Input: part model. Units: mm. Frame: model coordinates. Give positions to 0.01 mm unless a question says otherwise; leave off trailing zeros. Loops run counter-clockwise (first coordinate to the right, second up) from the corner with the lowest first, then second, coordinate; pieces in that order, holes last. Notation, with made-up numbers: (71, -0.75) - (112, -0.75) arc R28 cw to (112, 36.25) - close; hole circle Ø2 at (66.25, 49). An arc over 180 degrees is marked (long way). Answer as a JSON object with one key per item and string values. Group by question number.
(1) Pin query (flat end, axial travel): P1, Ø4.5, axis at x = 27.5, y = 0, coming from the +Z side. Return the tip coordinate at first contact, or that it passes through.
(2) Material intervals for L1, parallel to X at y = 0, z = 5.6; L2, parallel to Y at x = 27.5, z = 6.55; L3, parallel to Z at x = 26, y = -1, sorted ascending.
(3) Section query A-A (x = 27.5). Return loops of the section in (y, z).
(4) Section query B-B (y = 0). Return loops of the section in (x, z), plus the area to 3 significant figures.
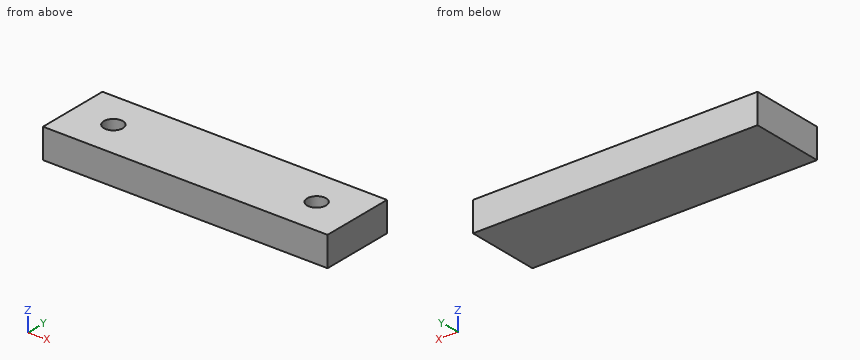
Autodesk Inventor part; units mm, degrees
ref_plane "YZ Plane" through (0, 0, 0) normal (1, 0, 0) x (0, 1, 0)
ref_plane "XZ Plane" through (0, 0, 0) normal (0, 1, 0) x (-1, 0, 0)
ref_plane "XY Plane" through (0, 0, 0) normal (0, 0, 1) x (1, 0, 0)
sketch "Sketch1" plane through (0, 0, 0) normal (0, 0, 1) x (1, 0, 0)
  line L0 (-38.5, -10) -> (38.5, -10)
  line L1 (38.5, -10) -> (38.5, 10)
  line L2 (38.5, 10) -> (-38.5, 10)
  line L3 (-38.5, 10) -> (-38.5, -10)
  line L4 (-38.5, -10) -> (38.5, 10) construction
  line L5 (38.5, -10) -> (-38.5, 10) construction
  point P0 (0, 0)
  dimension "d0" = 77
  dimension "d1" = 20
extrude "Extrusion1" add sketch "Sketch1" along normal blind 8
sketch "Sketch2" plane through (0, 0, 8) normal (0, 0, 1) x (1, 0, 0)
  line L0 (-38.5, -10) -> (38.5, -10)
  line L1 (38.5, -10) -> (38.5, 10)
  line L2 (-38.5, 10) -> (-38.5, -10)
  point P0 (0, 0)
  point P1 (-27.5, 0)
  point P2 (27.5, 0)
  point P3 (-38.5, 0)
  dimension "d4" = 10
  dimension "d5" = 10
  dimension "d6" = 11
  dimension "d14" = 11
hole "Hole1" at (-27.5, 0, 8) at (27.5, 0, 8) direction (0, 0, -1) diameter 5.134 depth 6
properties part number "Spann backe" material "Steel, Mild"
Recorded:
{
 "1": {"P1": "stops at z = 2"},
 "2": {"L1": "x = -38.5 to -30.07, -24.93 to 24.93, 30.07 to 38.5", "L2": "y = -10 to -2.57, 2.57 to 10", "L3": "z = 0 to 2"},
 "3": {"outline": "(-10, 0) - (10, 0) - (10, 8) - (2.57, 8) - (2.57, 2) - (-2.57, 2) - (-2.57, 8) - (-10, 8) - close"},
 "4": {"outline": "(-38.5, 0) - (38.5, 0) - (38.5, 8) - (30.07, 8) - (30.07, 2) - (24.93, 2) - (24.93, 8) - (-24.93, 8) - (-24.93, 2) - (-30.07, 2) - (-30.07, 8) - (-38.5, 8) - close", "area": "554 mm^2"}
}
